```python
from build123d import *

# Parameters (mm, degrees)
SKIZZE1_R                       = 12
AUFSATZ_LINEAR_AUSTRAGEN1_DEPTH = 15
SKIZZE2_R                       = 16.2
AUFSATZ_LINEAR_AUSTRAGEN3_DEPTH = 4
SKIZZE3_R                       = 6
SCHNITT_LINEAR_AUSTRAGEN1_DEPTH = 3
FASE1_SIZE                      = 1.5
FASE1_SIZE2                     = 2.598076211
SKIZZE4_R                       = 1.1
SCHNITT_LINEAR_AUSTRAGEN2_DEPTH = 16
SKIZZE5_R                       = 3
SCHNITT_LINEAR_AUSTRAGEN3_DEPTH = 3


with BuildPart() as part:
    # Skizze1 → Aufsatz-Linear austragen1 (new body)
    with BuildSketch(Plane.XY):
        with Locations((0, -12)):
            Circle(SKIZZE1_R)
    extrude(amount=AUFSATZ_LINEAR_AUSTRAGEN1_DEPTH)

    # Skizze2 → Aufsatz-Linear austragen3 (add)
    with BuildSketch(Plane.XY.offset(15)):
        with Locations((0, -12)):
            Circle(SKIZZE2_R)
    extrude(amount=-AUFSATZ_LINEAR_AUSTRAGEN3_DEPTH)

    # Skizze3 → Schnitt-Linear austragen1 (cut)
    with BuildSketch(Plane.XY):
        with Locations((0, -12)):
            Circle(SKIZZE3_R)
    extrude(amount=SCHNITT_LINEAR_AUSTRAGEN1_DEPTH, mode=Mode.SUBTRACT)

    # Fase1
    fase1_edges = [part.edges().sort_by_distance(p)[0] for p in [
        (-6, -12, 3),
    ]]
    fase1_side = [part.faces().sort_by_distance(p)[0] for p in [
        (0, -12, 3),
    ]]
    chamfer(fase1_edges, length=FASE1_SIZE, length2=FASE1_SIZE2, reference=fase1_side[0])

    # Skizze4 → Schnitt-Linear austragen2 (cut, through all)
    with BuildSketch(Plane.XY.offset(15)):
        with Locations((0, -12)):
            Circle(SKIZZE4_R)
    extrude(amount=-SCHNITT_LINEAR_AUSTRAGEN2_DEPTH, mode=Mode.SUBTRACT)

    # Skizze5 → Schnitt-Linear austragen3 (cut)
    with BuildSketch(Plane.XY.offset(15)):
        with Locations((0, -12)):
            Circle(SKIZZE5_R)
    extrude(amount=-SCHNITT_LINEAR_AUSTRAGEN3_DEPTH, mode=Mode.SUBTRACT)


solid = part.part
```
Can you work these out from the model? Positions are in its coordinate system, mm. A direction names the side the tool comes from. Round coordinates to 2 decimals unless told otherwise and drop trailing zeros. Loops run counter-clockwise (first coordinate to the right, second up) from the corner with the lowest first, then second, coordinate; pieces in that order, holes last. Notation, with made-up numbers: (71.5, 13.5) -> (125.5, 13.5) arc R33 ccw to (125.5, 46.5) -> close; hole circle Ø10 at (62, 11.5). An arc over 180 degrees is marked (long way). One line per item, written item: value. Start each with the question number.
1. For pin 1 (3 mm diameter, centred on x = -0.5, y = -11, fed in from +Z); pin 2 (3 mm diameter, centred on x = -11.5, z = 6.5, fed in from +Y); pin 3 (2.5 mm diameter, centred on x = -1, y = -11.5, fed in from -Z); pin 4 (19 mm diameter, centred on x = 0, y = -12, fed in from +Z), each with a flat end and sliding along its axis, tell me the tip position at first contact or that it passes through.
2. If we section it at B-B, the plane x = 0: Write out the boundary of the cut face in (y, z).
3. If we mould it in two halves opening along X, with no side actions, what happens to faces 4 (the cylindrical face through (-0.238, -13.074, 7.563)), 5 (the cylindrical face through (-2.601, -23.715, 5.423)), 6 (the flat face through (-11, -18, 11)), 7 (the cylindrical face through (-0.78, -6.05, 0.2))? For each: pulls with the +X half, pulls with the -X half, needs draft (parallel to the pull), parting line crosses it, or undercut.
4. If I drill on probe 1 along Y at (x, z) = (0, 13.4); probe 2 along Y at (x, z) = (0, 7); probe 3 along Z at (x, y) = (9, -23), over which ranges is the centre line in solid material (lowest first)?
5. If we section it at C-C, the plane z = 7.5: Write out the boundary of the cut face in (x, y).
6. If we section it at A-A, the plane y = -12: Write out the boundary of the cut face in (x, z).
7. If we section it at D-D, the plane x = 9: Write out the boundary of the cut face in (y, z).
8. For faces 1 (the flat face through (1, -13, 3)), 2 (the flat face through (0, -13.3, 12)), 3 (the cylindrical face through (8.71, 1.66, 13.03)), which set-ups out of +Z, -Z, +X, -X, +Y, -Y let a thin tool reach every point of the face, with its end or its side?
Calculated:
1. pin 1: stops at z = 12
1. pin 2: stops at y = -5.37
1. pin 3: stops at z = 3
1. pin 4: stops at z = 15
2. outline: (-28.2, 11) -> (-24, 11) -> (-24, 0) -> (-18, 0) -> (-18, 0.4) -> (-16.5, 3) -> (-13.1, 3) -> (-13.1, 12) -> (-15, 12) -> (-15, 15) -> (-28.2, 15) -> close; (-10.9, 3) -> (-7.5, 3) -> (-6, 0.4) -> (-6, 0) -> (0, 0) -> (0, 11) -> (4.2, 11) -> (4.2, 15) -> (-9, 15) -> (-9, 12) -> (-10.9, 12) -> close
3. face 4: undercut
3. face 5: parting line crosses it
3. face 6: needs draft
3. face 7: undercut
4. probe 1: y = -28.2 to -15, -9 to 4.2
4. probe 2: y = -24 to -13.1, -10.9 to 0
4. probe 3: z = 11 to 15
5. outline: circle Ø24 at (0, -12); hole circle Ø2.2 at (0, -12)
6. outline: (-16.2, 11) -> (-12, 11) -> (-12, 0) -> (-6, 0) -> (-6, 0.4) -> (-4.5, 3) -> (-1.1, 3) -> (-1.1, 12) -> (-3, 12) -> (-3, 15) -> (-16.2, 15) -> close; (1.1, 3) -> (4.5, 3) -> (6, 0.4) -> (6, 0) -> (12, 0) -> (12, 11) -> (16.2, 11) -> (16.2, 15) -> (3, 15) -> (3, 12) -> (1.1, 12) -> close
7. outline: (-25.47, 11) -> (-19.94, 11) -> (-19.94, 0) -> (-4.06, 0) -> (-4.06, 11) -> (1.47, 11) -> (1.47, 15) -> (-25.47, 15) -> close
8. face 1: -Z
8. face 2: +Z
8. face 3: +Z, -Z
